Work out the finished part from the listing and answer in its coordinate system (mm). A direction names the side the tool comes from. Round coordinates to 2 decimals unless told otherwise and drop trailing zeros. Write each loop counter-clockwise with the first axis right and the second up, starting at its lowest first coordinate (ties: lowest second). Pieces come first, ordered by that corner, then holes. Notation, with made-up numbers: (51, 44) -> (70, 44) arc R24 ccw to (70, 75) -> close; hole circle Ø9 at (14.25, -35.75). An arc over 180 degrees is marked (long way). One line per item, written item: value.
```python
from build123d import *

# Parameters (mm, degrees)
SKETCH1_W           = 45
SKETCH1_H           = 15
BOSS_EXTRUDE1_DEPTH = 9.5
SKETCH2_R           = 5.5
CUT_EXTRUDE1_DEPTH  = 8
CUT_EXTRUDE6_DEPTH  = 8
CUT_EXTRUDE2_REACH  = 3.5
SKETCH4_R           = 2.175
CUT_EXTRUDE3_DEPTH  = 2
FILLET1_R           = 7
SKETCH5_R           = 2.05
CUT_EXTRUDE4_DEPTH  = 5
SKETCH6_R           = 0.95
CUT_EXTRUDE5_DEPTH  = 3
FILLET3_R           = 1


with BuildPart() as part:
    # Sketch1 → Boss-Extrude1 (new body)
    with BuildSketch(Plane(origin=(0, 0, 0), x_dir=(1, 0, 0), z_dir=(0, 1, 0))):
        with Locations((22.5, 7.5)):
            Rectangle(SKETCH1_W, SKETCH1_H)
    extrude(amount=-BOSS_EXTRUDE1_DEPTH)

    # Sketch2 → Cut-Extrude1 (cut)
    with BuildSketch(Plane(origin=(0, 0, 0), x_dir=(1, 0, 0), z_dir=(0, 1, 0))):
        with Locations((22.5, 8.82)):
            Circle(SKETCH2_R)
    extrude(amount=-CUT_EXTRUDE1_DEPTH, mode=Mode.SUBTRACT)

    # Sketch8 → Cut-Extrude6 (cut)
    with BuildSketch(Plane(origin=(0, 0, 0), x_dir=(1, 0, 0), z_dir=(0, 1, 0))):
        with BuildLine():
            Line((16.85, 8.85), (16.85, 6.15))
            ThreePointArc((16.85, 6.15), (22.5, 0.5), (28.15, 6.15))
            Line((28.15, 6.15), (28.15, 8.85))
            ThreePointArc((28.15, 8.85), (22.5, 14.5), (16.85, 8.85))
        make_face()
    extrude(amount=-CUT_EXTRUDE6_DEPTH, mode=Mode.SUBTRACT)

    # Sketch3 → Cut-Extrude2 (cut, up to next)
    with BuildSketch(Plane(origin=(0, -8, 0), x_dir=(1, 0, 0), z_dir=(0, 1, 0)), mode=Mode.PRIVATE) as cut_extrude2_sk1:
        with BuildLine():
            Line((20, 11.5), (20, 3.5))
            ThreePointArc((20, 3.5), (22.5, 1), (25, 3.5))
            Line((25, 3.5), (25, 11.5))
            ThreePointArc((25, 11.5), (22.5, 14), (20, 11.5))
        make_face()
    cut_extrude2_tool1 = extrude(cut_extrude2_sk1.sketch, amount=-CUT_EXTRUDE2_REACH, mode=Mode.PRIVATE) & part.part
    add(cut_extrude2_tool1.solids().sort_by_distance((22.5, -8, -7.5))[0], mode=Mode.SUBTRACT)

    # Sketch4 → Cut-Extrude3 (cut)
    with BuildSketch(Plane(origin=(0, 0, 0), x_dir=(1, 0, 0), z_dir=(0, 1, 0))):
        with Locations((6, 7.5)):
            Circle(SKETCH4_R)
        with Locations((39, 7.5)):
            Circle(SKETCH4_R)
    extrude(amount=-CUT_EXTRUDE3_DEPTH, mode=Mode.SUBTRACT)

    # Fillet1
    fillet1_edges = [part.edges().sort_by_distance(p)[0] for p in [
        (0, -4.75, -15),
        (45, -4.75, -15),
        (45, -4.75, 0),
        (0, -4.75, 0),
    ]]
    fillet(fillet1_edges, radius=FILLET1_R)

    # Sketch5 → Cut-Extrude4 (cut)
    with BuildSketch(Plane(origin=(0, -9.5, 0), x_dir=(-1, 0, 0), z_dir=(0, -1, 0))):
        with Locations((-39, 7.5)):
            Circle(SKETCH5_R)
        with Locations((-6, 7.5)):
            Circle(SKETCH5_R)
    extrude(amount=-CUT_EXTRUDE4_DEPTH, mode=Mode.SUBTRACT)

    # Sketch6 → Cut-Extrude5 (cut)
    with BuildSketch(Plane(origin=(0, -2, 0), x_dir=(1, 0, 0), z_dir=(0, 1, 0))):
        with Locations((6, 7.5)):
            Circle(SKETCH6_R)
        with Locations((39, 7.5)):
            Circle(SKETCH6_R)
    extrude(amount=-CUT_EXTRUDE5_DEPTH, mode=Mode.SUBTRACT)

    # Fillet3
    fillet3_edges = [part.edges().sort_by_distance(p)[0] for p in [
        (22.5, -8, -14),
        (20, -8, -7.5),
        (22.5, -8, -1),
        (25, -8, -7.5),
    ]]
    fillet(fillet3_edges, radius=FILLET3_R)


solid = part.part
```
(1) Flat-ended cylindrical pins translate along their axes: pin 1 Ø3 at (x, z) = (39, -7.5) entering from +Y; pin 2 Ø8 at (x, z) = (22, -9) entering from +Y; pin 3 Ø2 at (x, z) = (39.5, -7) entering from -Y. Find the tip coordinate at first contact, or state that the pin passes through.
Reported:
pin 1: stops at y = -2
pin 2: stops at y = -8
pin 3: stops at y = -4.5
(2) A tool of negligible diameter and unlimited length cuts with its end or side. For faces 1 (the face through (8.05, -7.04, -7.59)), 2 (the face through (28.15, -4, -7)), 3 (the face through (42.9, -4.8, -2)), from which of +Z, -Z, +X, -X, +Y, -Y can it reach the whole face along a straight path? Write none if from no direction.
Reported:
face 1: -Y
face 2: +Y
face 3: +Z, +X, +Y, -Y
(3) Find section A-A on y = -7. Give the vertices of the cut face in (x, z).
Reported:
outline: (0, -8) arc R7 ccw to (7, -15) -> (38, -15) arc R7 ccw to (45, -8) -> (45, -7) arc R7 ccw to (38, 0) -> (7, 0) arc R7 ccw to (0, -7) -> close; hole circle Ø4.1 at (6, -7.5); hole (16.85, -8.85) arc R5.65 ccw to (28.15, -8.85) -> (28.15, -6.15) arc R5.65 ccw to (16.85, -6.15) -> close; hole circle Ø4.1 at (39, -7.5)
(4) For a pull along Z with two mould halves and no side action, classify faces 4 (the face through (45, -4.7, -7.5)), 5 (the face through (16.85, -4, -8)), 6 (the face through (22, -5, -15)) as pulls with the +Z half, pulls with the -Z half, needs draft (parallel to the pull), parting line crosses it, or undercut.
Reported:
face 4: needs draft
face 5: undercut
face 6: pulls with the -Z half
(5) Find section B-B on x = 6. Give the vertices of the cut face in (y, z) (3 decimals).
Reported:
outline: (-9.5, -14.928) -> (0, -14.928) -> (0, -9.675) -> (-2, -9.675) -> (-2, -8.45) -> (-4.5, -8.45) -> (-4.5, -9.55) -> (-9.5, -9.55) -> close; (-9.5, -5.45) -> (-4.5, -5.45) -> (-4.5, -6.55) -> (-2, -6.55) -> (-2, -5.325) -> (0, -5.325) -> (0, -0.072) -> (-9.5, -0.072) -> close
(6) Find section D-D on z = -7.5. Give the number of separate pieces and of enclosed holes in the cut face, plus the area to 3 significant figures.
Reported:
separate pieces: 4
enclosed holes: 0
area: 261 mm2
(7) Find section C-C on z = -4.75. Give the vertices of the cut face in (x, y), plus the area to 3 significant figures.
Reported:
outline: (0.37, -9.5) -> (20, -9.5) -> (20, -9) arc R1 ccw to (19, -8) -> (17.03, -8) -> (17.03, 0) -> (0.37, 0) -> close; (25, -9.5) -> (44.63, -9.5) -> (44.63, 0) -> (27.97, 0) -> (27.97, -8) -> (26, -8) arc R1 ccw to (25, -9) -> close
area: 325 mm2
(8) Consider probe 1 along X at (y, z) = (-5.55, -7.5); probe 2 along X at (y, z) = (-2.9, -7.5); probe 3 along X at (y, z) = (-5, -13.75). Determine where each line is inside the solid, lowest interval first.
Reported:
probe 1: x = 0 to 3.95, 8.05 to 16.85, 28.15 to 36.95, 41.05 to 45
probe 2: x = 0 to 5.05, 6.95 to 16.85, 28.15 to 38.05, 39.95 to 45
probe 3: x = 3.01 to 19.69, 25.31 to 41.99
